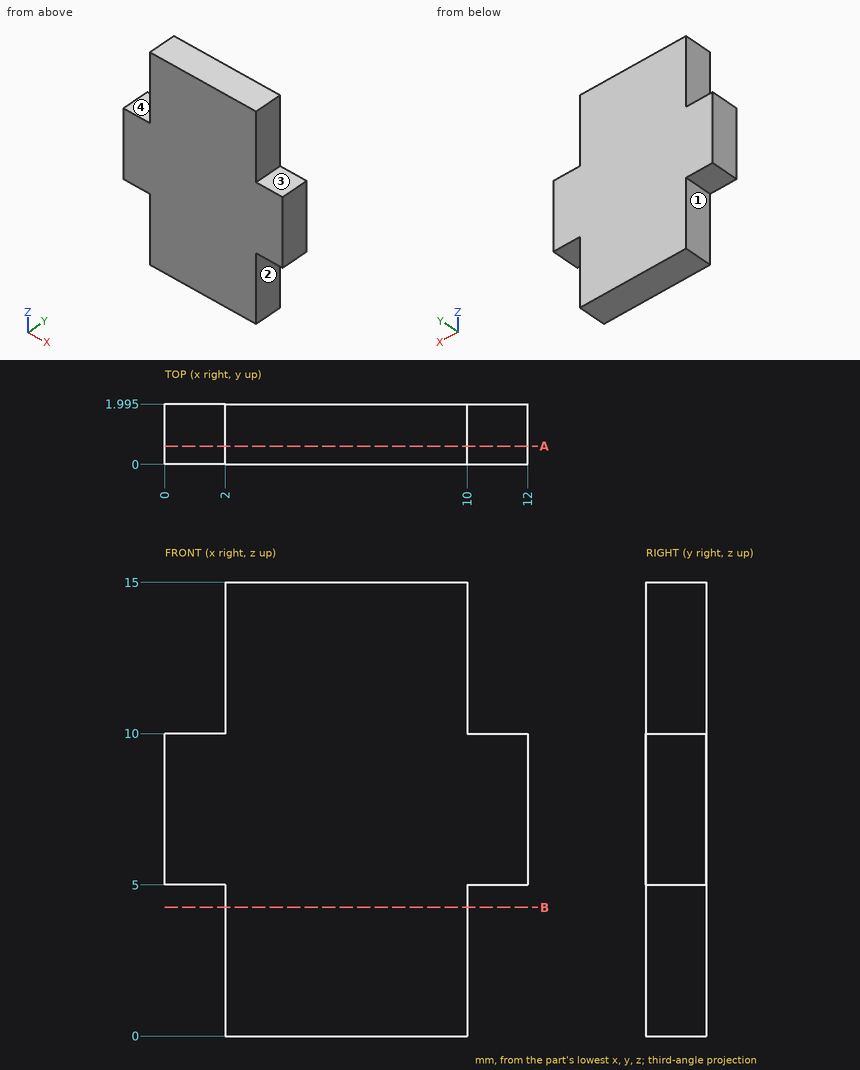
Verification items for this drawing (mm, ordinates from the low corner). A direction names the side the tool comes from. Give positions to 0.01 mm unless a question says otherwise; leave off trailing zeros. Write each loop counter-clockwise with the first axis right and the second up, starting at its lowest first coordinate (ties: lowest second). Pieces come first, ordered by that corner, then holes.
1) Material ranges on L1, parallel to Z at x = 10.5, y = 0.95; L2, parallel to X at y = 1, z = 4.5, recorded low to high.
2) Section check B-B, the plane z = 4.25. Record the boundary of the cut face in (x, y) (1 decimal).
3) Gauge pin test, flat ends, axial feed: pin 1 (1 mm diameter, centred on y = 0.5, z = 12.5, fed in from +X); pin 2 (0.6 mm diameter, centred on x = 11.5, y = 1, fed in from -Z); pin 3 (0.6 mm diameter, centred on x = 11.5, y = 0.5, fed in from +Z). Record the tip position at first contact, or that the pin passes through.
4) Access from +Z, -Z, +X, -X, +Y, -Y to the whole of each face (thin tool, end or side, straight path). Record for the marked faces 1, 2, 3 and 4.
5) Section check A-A, the plane y = 0.6. Record the boundary of the cut face in (x, z), and give its area (3 significant figures).
Computed:
1. L1: z = 5 to 10
1. L2: x = 2 to 10
2. outline: (2, 0) - (10, 0) - (10, 2) - (2, 2) - close
3. pin 1: stops at x = 10
3. pin 2: stops at z = 5
3. pin 3: stops at z = 10
4. face 1: -Z, -X, +Y, -Y
4. face 2: -Z, +X, +Y, -Y
4. face 3: +Z, +X, +Y, -Y
4. face 4: +Z, -X, +Y, -Y
5. outline: (0, 5) - (2, 5) - (2, 0) - (10, 0) - (10, 5) - (12, 5) - (12, 10) - (10, 10) - (10, 15) - (2, 15) - (2, 10) - (0, 10) - close
5. area: 140 mm2
